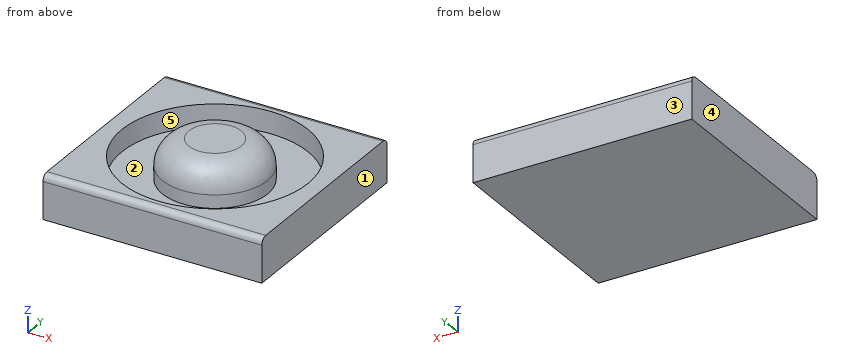
```python
from build123d import *

# Parameters (mm, degrees)
F0_W     = 100
F0_H     = 95
F1_DEPTH = 10
F2_R     = 42.5
F2_R_2   = 24
F3_DEPTH = 10
F4_R     = 24
F4_R_2   = 14
F5_DEPTH = 8
F6_R     = 12
F7_R     = 3


with BuildPart() as f1:
    # F0 (on Top) → F1 (new body, symmetric)
    with BuildSketch(Plane.XY):
        Rectangle(F0_W, F0_H)
    extrude(amount=F1_DEPTH, both=True)

    # F2 (on face) → F3 (cut)
    with BuildSketch(Plane.XY.offset(10)):
        Circle(F2_R)
        Circle(F2_R_2, mode=Mode.SUBTRACT)
    extrude(amount=-F3_DEPTH, mode=Mode.SUBTRACT)

    # F4 (on face) → F5 (join)
    with BuildSketch(Plane.XY.offset(10)):
        Circle(F4_R)
        Circle(F4_R_2, mode=Mode.SUBTRACT)
        Circle(F4_R_2)
    extrude(amount=F5_DEPTH)

    # F6
    f6_edges = [f1.edges().sort_by_distance(p)[0] for p in [
        (-24, 0, 18),
    ]]
    fillet(f6_edges, radius=F6_R)

    # F7
    f7_edges = [f1.edges().sort_by_distance(p)[0] for p in [
        (0, 47.5, 10),
        (0, -47.5, 10),
    ]]
    fillet(f7_edges, radius=F7_R)


solid = f1.part
```
Geometry check sheet. Reference: the model listing, model coordinates, mm. Face numbers are marked on the shaded views. A direction names the side the tool comes from. Round coordinates to 2 decimals unless told otherwise and drop trailing zeros. Loops run counter-clockwise (first coordinate to the right, second up) from the corner with the lowest first, then second, coordinate; pieces in that order, holes last. Notation, with made-up numbers: (10.25, 4.5) - (51.25, 4.5) arc R20 ccw to (51.25, 23.5) - close; hole circle Ø3 at (18.25, 35.5). An arc over 180 degrees is marked (long way). Use a Markdown table: item, result.
Q1. Cross-section at D-D on x = -30. Record the cut outline in (y, z), plus the area to 3 significant figures.
Solutions:
| item | result |
|---|---|
| outline | (-47.5, -10) - (47.5, -10) - (47.5, 7) arc R3 ccw to (44.5, 10) - (30.1, 10) - (30.1, 0) - (-30.1, 0) - (-30.1, 10) - (-44.5, 10) arc R3 ccw to (-47.5, 7) - close |
| area | 1,290 mm2 |
Q2. Access from +Z, -Z, +X, -X, +Y, -Y to the whole of each face (thin tool, end or side, straight path). Record for the marked faces 4 and 5.
Solutions:
| item | result |
|---|---|
| face 4 | +Z, -Z, -X, +Y, -Y |
| face 5 | +Z |
Q3. Cross-section at A-A on z = 4.5. Record the cut outline in (x, y), plus the area to 3 significant figures.
Solutions:
| item | result |
|---|---|
| outline | (-50, -47.5) - (50, -47.5) - (50, 47.5) - (-50, 47.5) - close; circle Ø48 at (0, 0); hole circle Ø85 at (0, 0) |
| area | 5,640 mm2 |
Q4. Cross-section at C-C on y = 26.5. Record the cut outline in (x, z), plus the area to 3 significant figures.
Solutions:
| item | result |
|---|---|
| outline | (-50, -10) - (50, -10) - (50, 10) - (33.23, 10) - (33.23, 0) - (-33.23, 0) - (-33.23, 10) - (-50, 10) - close |
| area | 1,340 mm2 |
Q5. Go/stop test with flat-tipped pins: P1, Ø10, axis at y = -14.5, z = 13.5, coming from the +X side; P2, Ø5, axis at x = 1.5, y = -33.5, coming from the +Z side. Record where each tip stops, or that it passes through.
Solutions:
| item | result |
|---|---|
| P1 | stops at x = 50 |
| P2 | stops at z = 0 |
Q6. Cross-section at B-B on x = 38.5. Record the cut outline in (y, z), plus the area to 3 significant figures.
Solutions:
| item | result |
|---|---|
| outline | (-47.5, -10) - (47.5, -10) - (47.5, 7) arc R3 ccw to (44.5, 10) - (18, 10) - (18, 0) - (-18, 0) - (-18, 10) - (-44.5, 10) arc R3 ccw to (-47.5, 7) - close |
| area | 1,540 mm2 |
Q7. Material ranges on line 1 (Y direction, x = 0, z = 5); line 2 (X direction, y = -19.5, z = 6); line 3 (X direction, y = -22, z = 5), recorded low to high.
Solutions:
| item | result |
|---|---|
| line 1 | y = -47.5 to -42.5, -24 to 24, 42.5 to 47.5 |
| line 2 | x = -50 to -37.76, -13.99 to 13.99, 37.76 to 50 |
| line 3 | x = -50 to -36.36, -9.59 to 9.59, 36.36 to 50 |
Q8. Draft check along X on the marked faces 1, 2 and 3. Enter one of: released by +X, released by -X, zero draft, split by the parting line, or undercut.
Solutions:
| item | result |
|---|---|
| face 1 | released by +X |
| face 2 | undercut |
| face 3 | zero draft |
